Geometry check sheet. Reference: the model listing, model coordinates, mm. A direction names the side the tool comes from. Give positions to 0.01 mm unless a question says otherwise; leave off trailing zeros. Write each loop counter-clockwise with the first axis right and the second up, starting at its lowest first coordinate (ties: lowest second). Pieces come first, ordered by that corner, then holes. Notation, with made-up numbers: (30, 10.5) - (58, 10.5) arc R15 ccw to (58, 28.5) - close; hole circle Ø9 at (-39.75, 77.5). An arc over 180 degrees is marked (long way). Write item = value, one per line. Start each with the question number.
(1) Section check C-C, the plane z = 0. Enter the section's corners in (x, y), plus the area to 3 significant figures.
(2) Section check A-A, the plane y = 0. Enter the section's corners in (x, z).
(3) Thickness scan on L1, parallel to X at y = 0, z = 1.45; L2, parallel to X at y = 0, z = 1.35; L3, parallel to Y at x = 0, z = 1.15. Record the ranges inside material, lowest first.
(4) Depth check by flat-ended pin: pin 1 Ø1 at (x, y) = (-0.5, -3) entering from +Z; pin 2 Ø1.5 at (x, z) = (-2.5, -1) entering from +Y; pin 3 Ø2.5 at (x, y) = (0, 0) entering from -Z. Enter the tip coordinate at first touch or a pass-through.
(5) Access from +Z, -Z, +X, -X, +Y, -Y to the whole of each face (thin tool, end or side, straight path). Record for faces 1 (the flat face through (-2, 2, -2)), 2 (the flat face through (2, 2, 1)), 3 (the flat face through (0, 4, -2.5)).
(6) Draft check along X on faces 4 (the cylindrical face through (-0.29, -2.23, -2.25)), 5 (the flat face through (-2, 0, 1.5)), 6 (the cylindrical face through (-0.59, -4.46, -0.48)). Enter one of: pulls with the +X half, pulls with the -X half, needs draft (parallel to the pull), parting line crosses it, or undercut.
```python
from build123d import *


with BuildPart() as part:
    # Sketch1 → Revolve1 (revolve)
    with BuildSketch(Plane.XZ):
        Polygon((4.5, 1.25), (4.25, 1.5), (3.75, 1.5), (3.75, 1), (2.25, 1), (2.25, 1.5), (1.5, 1.5), (1.5, -2.5), (2.25, -2.5), (2.25, -2), (3.75, -2), (3.75, -2.5), (4.25, -2.5), (4.5, -2.25), align=None)
    revolve(axis=Axis((0, 0, 2.5), (0, 0, -1)))


solid = part.part
```
Model answer:
q1.outline = circle Ø9 at (0, 0); hole circle Ø3 at (0, 0)
q1.area = 56.5 mm²
q2.outline = (-4.5, -2.25) - (-4.25, -2.5) - (-3.75, -2.5) - (-3.75, -2) - (-2.25, -2) - (-2.25, -2.5) - (-1.5, -2.5) - (-1.5, 1.5) - (-2.25, 1.5) - (-2.25, 1) - (-3.75, 1) - (-3.75, 1.5) - (-4.25, 1.5) - (-4.5, 1.25) - close; (1.5, -2.5) - (2.25, -2.5) - (2.25, -2) - (3.75, -2) - (3.75, -2.5) - (4.25, -2.5) - (4.5, -2.25) - (4.5, 1.25) - (4.25, 1.5) - (3.75, 1.5) - (3.75, 1) - (2.25, 1) - (2.25, 1.5) - (1.5, 1.5) - close
q3.L1 = -4.3 to -3.75, -2.25 to -1.5, 1.5 to 2.25, 3.75 to 4.3
q3.L2 = -4.4 to -3.75, -2.25 to -1.5, 1.5 to 2.25, 3.75 to 4.4
q3.L3 = -4.5 to -3.75, -2.25 to -1.5, 1.5 to 2.25, 3.75 to 4.5
q4.pin_1 = 1
q4.pin_2 = 4.15
q4.pin_3 = through
q5.face_1 = -Z
q5.face_2 = +Z
q5.face_3 = -Z, +X, -X, +Y, -Y
q6.face_4 = undercut
q6.face_5 = needs draft
q6.face_6 = parting line crosses it
